from build123d import *

# Parameters (mm, degrees)
F0_W     = 70
F0_H     = 50
F1_DEPTH = 50
F2_W     = 50
F2_H     = 20
F3_DEPTH = 30
F4_W     = 50
F4_H     = 10
F5_DEPTH = 30
F6_W     = 20
F6_H     = 20
F7_DEPTH = 20
F8_SIZE  = 10


with BuildPart() as f1:
    # F0 (on Top) → F1 (new body)
    with BuildSketch(Plane.XY):
        with Locations((35, 25)):
            Rectangle(F0_W, F0_H)
    extrude(amount=F1_DEPTH)

    # F2 (on face) → F3 (cut)
    with BuildSketch(Plane.XY.offset(50)):
        with Locations((45, 10)):
            Rectangle(F2_W, F2_H)
    extrude(amount=-F3_DEPTH, mode=Mode.SUBTRACT)

    # F4 (on face) → F5 (cut)
    with BuildSketch(Plane.XY.offset(50)):
        with Locations((45, 45)):
            Rectangle(F4_W, F4_H)
    extrude(amount=-F5_DEPTH, mode=Mode.SUBTRACT)

    # F6 (on face) → F7 (cut, through all)
    with BuildSketch(Plane.XZ.offset(-20)):
        with Locations((30, 30)):
            Rectangle(F6_W, F6_H)
    extrude(amount=-F7_DEPTH, mode=Mode.SUBTRACT)

    # F8
    f8_edges = [f1.edges().sort_by_distance(p)[0] for p in [
        (70, 0, 10),
    ]]
    chamfer(f8_edges, length=F8_SIZE)


solid = f1.part
Source: CAD feature listing. Evaluate the final solid. Frame: model axes, mm. A direction names the side the tool comes from. Round coordinates to 2 decimals unless told otherwise and drop trailing zeros. Loops run counter-clockwise (first coordinate to the right, second up) from the corner with the lowest first, then second, coordinate; pieces in that order, holes last. Notation, with made-up numbers: (46.25, 44) - (62.25, 44) arc R18 cw to (62.25, 66) - close; hole circle Ø10 at (64, 56.5). An arc over 180 degrees is marked (long way). Write item = value, one per line. Start each with the question number.
Item 1: Section query C-C on x = 37.5. Output: boundary loops of the cut face in (y, z), plus the area to 3 significant figures.
Item 2: First-contact query: pin 1 Ø8 at (x, y) = (46.5, 17) entering from -Z; pin 2 Ø15 at (x, z) = (52, 38.5) entering from -Y; pin 3 Ø15 at (x, z) = (34.5, 35.5) entering from +Y; pin 4 Ø5 at (y, z) = (6.5, 38.5) entering from +X. Flat tips, straight axial feed; report the tip coordinate or a pass-through.
Item 3: Section query B-B on z = 33. Output: boundary loops of the cut face in (x, y).
Item 4: Reachability of faces 4 (the face through (39, 25, 20)), 5 (the face through (50, 40, 39)), 6 (the face through (50, 20, 39)), 7 (the face through (35, 25, 0)), 8 (the face through (30, 30, 40)) from +Z, -Z, +X, -X, +Y, -Y: full face, straight path, thin tool, end or side. Return the list, or none.
Item 5: Material intervals for line 1 (Z direction, x = 27.5, y = 38.5); line 2 (X direction, y = 27, z = 23.5); line 3 (Z direction, x = 50, y = 15.5), sorted ascending.
Item 6: Mould query, pull axis Z, two halves, no side actions, for faces 1 (the face through (27, 25, 50)), 2 (the face through (20, 25, 35)), 3 (the face through (27, 50, 19)). Classes: released by +Z, released by -Z, zero draft, split by the parting line, or undercut.
Item 7: Section query A-A on y = 22. Output: boundary loops of the cut face in (x, z).
Item 8: Section query D-D on z = 41.5. Output: boundary loops of the cut face in (x, y).
Results list:
q1.outline = (0, 0) - (50, 0) - (50, 20) - (0, 20) - close; (20, 40) - (40, 40) - (40, 50) - (20, 50) - close
q1.area = 1,200 mm²
q2.pin_1 = 0
q2.pin_2 = 20
q2.pin_3 = 40
q2.pin_4 = 20
q3.outline = (0, 0) - (20, 0) - (20, 50) - (0, 50) - close; (40, 20) - (70, 20) - (70, 40) - (40, 40) - close
q4.face_4 = none
q4.face_5 = +Z, +X, +Y
q4.face_6 = +Z, +X, -Y
q4.face_7 = -Z, +X, -X, +Y, -Y
q4.face_8 = +Y, -Y
q5.line_1 = 0 to 20, 40 to 50
q5.line_2 = 0 to 20, 40 to 70
q5.line_3 = 0 to 20
q6.face_1 = released by +Z
q6.face_2 = undercut
q6.face_3 = zero draft
q7.outline = (0, 0) - (70, 0) - (70, 50) - (0, 50) - close; hole (20, 20) - (40, 20) - (40, 40) - (20, 40) - close
q8.outline = (0, 0) - (20, 0) - (20, 20) - (70, 20) - (70, 40) - (20, 40) - (20, 50) - (0, 50) - close
